Source: CAD feature listing. Evaluate the final solid. Frame: model axes, mm. A direction names the side the tool comes from. Round coordinates to 2 decimals unless told otherwise and drop trailing zeros. Write each loop counter-clockwise with the first axis right and the second up, starting at its lowest first coordinate (ties: lowest second). Pieces come first, ordered by that corner, then holes.
from build123d import *

# Parameters (mm, degrees)
SKETCH1_W           = 25.4
SKETCH1_H           = 2.286
BOSS_EXTRUDE1_DEPTH = 4.064
SKETCH3_W           = 25.4
SKETCH3_H           = 2.54
BOSS_EXTRUDE3_DEPTH = 7.112
SKETCH4_W           = 0.762
SKETCH4_H           = 1.016
CUT_EXTRUDE1_DEPTH  = 30.734


with BuildPart() as part:
    # Sketch1 → Boss-Extrude1 (new body)
    with BuildSketch(Plane(origin=(0, 0, 0), x_dir=(1, 0, 0), z_dir=(0, 1, 0))):
        with Locations((-2.386060606, 1.550939394)):
            Rectangle(SKETCH1_W, SKETCH1_H)
    extrude(amount=BOSS_EXTRUDE1_DEPTH)

    # Sketch3 → Boss-Extrude3 (add)
    with BuildSketch(Plane(origin=(0, 0, -2.693939394), x_dir=(-1, 0, 0), z_dir=(0, 0, -1))):
        with Locations((2.386060606, 0.254)):
            Rectangle(SKETCH3_W, SKETCH3_H)
    extrude(amount=BOSS_EXTRUDE3_DEPTH)

    # Sketch4 → Cut-Extrude1 (cut)
    with BuildSketch(Plane.ZY.offset(15.086060606)):
        with Locations((-3.074939394, -0.508)):
            Rectangle(SKETCH4_W, SKETCH4_H)
    extrude(amount=-CUT_EXTRUDE1_DEPTH, mode=Mode.SUBTRACT)


solid = part.part
1) Section query A-A on x = -6.25. Return the cut outline in (y, z), then the cut area to 3 significant figures.
Taken from the geometry:
outline: (-1.02, -9.81) - (1.52, -9.81) - (1.52, -2.69) - (4.06, -2.69) - (4.06, -0.41) - (0, -0.41) - (0, -3.46) - (-1.02, -3.46) - close
area: 26.6 mm2
2) Contact query for flat-ended pins moving along their axis: P1, Ø2, axis at x = 2.5, z = -5.5, coming from the +Y side; P2, Ø1.3, axis at x = 3.5, y = 2.5, coming from the -Z side. Output: stop coordinate, or through.
Taken from the geometry:
P1: stops at y = 1.52
P2: stops at z = -2.69
3) Section query C-C on z = -5. Return the cut outline in (x, y), then the cut area to 3 significant figures.
Taken from the geometry:
outline: (-15.09, -1.02) - (10.31, -1.02) - (10.31, 1.52) - (-15.09, 1.52) - close
area: 64.5 mm2
4) Reachability of faces 1 (the face through (-3, 0, -2)), 2 (the face through (-2, 0, -9.806)), 3 (the face through (-3, 3, -2.694)) from +Z, -Z, +X, -X, +Y, -Y: full face, straight path, thin tool, end or side. Return the list, or none.
Taken from the geometry:
face 1: +Z, +X, -X, -Y
face 2: -Z, +X, -X, +Y, -Y
face 3: -Z, +X, -X, +Y
5) Section query B-B on y = 2.5. Return the cut outline in (x, z), then the cut area to 3 significant figures.
Taken from the geometry:
outline: (-15.09, -2.69) - (10.31, -2.69) - (10.31, -0.41) - (-15.09, -0.41) - close
area: 58.1 mm2
6) Material intervals for line 1 (Z direction, x = -7.25, y = 2.5); line 2 (Y direction, x = 5.5, z = -7.25); line 3 (Y direction, x = -11.5, z = -1.25), sorted ascending.
Taken from the geometry:
line 1: z = -2.69 to -0.41
line 2: y = -1.02 to 1.52
line 3: y = 0 to 4.06
